```python
from build123d import *

# Parameters (mm, degrees)
BASE_FLANGE1_DEPTH     = 2
TAB1_START             = -2
TAB1_OUTLINE_W         = 950
TAB1_OUTLINE_H         = 35
TAB1_DEPTH             = 2
SKETCHED_START         = -950
SKETCHED_BEND1_DEPTH   = 950
SKETCHED_BEND1_2_DEPTH = 950
FILLET1_R              = 0.78
FILLET2_R              = 0.74
SKETCH10_R             = 12.5
SKETCH10_R_2           = 22.5
CUT_EXTRUDE1_DEPTH     = 10
SKETCH11_R             = 4
CUT_EXTRUDE2_DEPTH     = 10
SKETCH12_R             = 12.5
CUT_EXTRUDE3_DEPTH     = 10


# Read off the part's stored shape, not the designer's step: Tab1, Sketched Bend1
# Sheet-metal steps are written as plain solids
with BuildPart() as part:
    # Sketch1 → Base-Flange1 (new body)
    with BuildSketch(Plane(origin=(0, 0, 0), x_dir=(0, 0, -1), z_dir=(1, 0, 0))):
        Polygon((0, 0), (0, -300), (650, -550), (950, -550), (950, 0), align=None)
    extrude(amount=-BASE_FLANGE1_DEPTH)

    # Tab1 outline → Tab1 (add)
    with BuildSketch(Plane(origin=(0, 0, 0), x_dir=(0, 0, -1), z_dir=(1, 0, 0)).offset(TAB1_START)):
        with Locations((475, 17.5)):
            Rectangle(TAB1_OUTLINE_W, TAB1_OUTLINE_H)
    extrude(amount=TAB1_DEPTH)

    # Sketched Bend1 outline → Sketched Bend1 (cut)
    with BuildSketch(Plane.XY.offset(SKETCHED_START)):
        with BuildLine():
            ThreePointArc((-2, 0), (-1.443395312, 1.654267209), (0, 2.635602398))
            Line((0, 2.635602398), (0, 35))
            Line((0, 35), (-2, 35))
            Line((-2, 35), (-2, 0))
        make_face()
    extrude(amount=SKETCHED_BEND1_DEPTH, mode=Mode.SUBTRACT)

    # Sketched Bend1 2 outline → Sketched Bend1 2 (add)
    with BuildSketch(Plane.XY.offset(SKETCHED_START)):
        with BuildLine():
            Line((33.008755099, 2.7366), (0.7366, 2.7366))
            ThreePointArc((0.7366, 2.7366), (0.364854094, 2.711233029), (0, 2.635602398))
            Line((0, 2.635602398), (0, 0))
            ThreePointArc((0, 0), (0.215745145, 0.520854855), (0.7366, 0.7366))
            Line((0.7366, 0.7366), (33.008755099, 0.7366))
            Line((33.008755099, 0.7366), (33.008755099, 2.7366))
        make_face()
    extrude(amount=SKETCHED_BEND1_2_DEPTH)

    # Fillet1
    fillet1_edges = [part.edges().sort_by_distance(p)[0] for p in [
        (-1, -300, 0),
    ]]
    fillet(fillet1_edges, radius=FILLET1_R)

    # Fillet2
    fillet2_edges = [part.edges().sort_by_distance(p)[0] for p in [
        (-1, -550, -650),
    ]]
    fillet(fillet2_edges, radius=FILLET2_R)

    # Sketch10 → Cut-Extrude1 (cut)
    with BuildSketch(Plane(origin=(0, 0, 0), x_dir=(0, 0, -1), z_dir=(1, 0, 0))):
        with Locations((800.068700733, -27.5)):
            Circle(SKETCH10_R)
        with Locations((800.068700733, -522.5)):
            Circle(SKETCH10_R_2)
    extrude(amount=-CUT_EXTRUDE1_DEPTH, mode=Mode.SUBTRACT)

    # Sketch11 → Cut-Extrude2 (cut)
    with BuildSketch(Plane.XZ.offset(-0.7366)):
        with Locations((16.872677549, -25)):
            Circle(SKETCH11_R)
        with Locations((16.872677549, -125)):
            Circle(SKETCH11_R)
        with Locations((16.872677549, -225)):
            Circle(SKETCH11_R)
        with Locations((16.872677549, -325)):
            Circle(SKETCH11_R)
        with Locations((16.872677549, -425)):
            Circle(SKETCH11_R)
        with Locations((16.872677549, -525)):
            Circle(SKETCH11_R)
        with Locations((16.872677549, -625)):
            Circle(SKETCH11_R)
        with Locations((16.872677549, -725)):
            Circle(SKETCH11_R)
        with Locations((16.872677549, -825)):
            Circle(SKETCH11_R)
        with Locations((16.872677549, -925)):
            Circle(SKETCH11_R)
    extrude(amount=-CUT_EXTRUDE2_DEPTH, mode=Mode.SUBTRACT)

    # Sketch12 → Cut-Extrude3 (cut)
    with BuildSketch(Plane(origin=(0, 0, 0), x_dir=(0, 0, -1), z_dir=(1, 0, 0))):
        with Locations((125, -97.2634)):
            Circle(SKETCH12_R)
    extrude(amount=-CUT_EXTRUDE3_DEPTH, mode=Mode.SUBTRACT)


solid = part.part
```
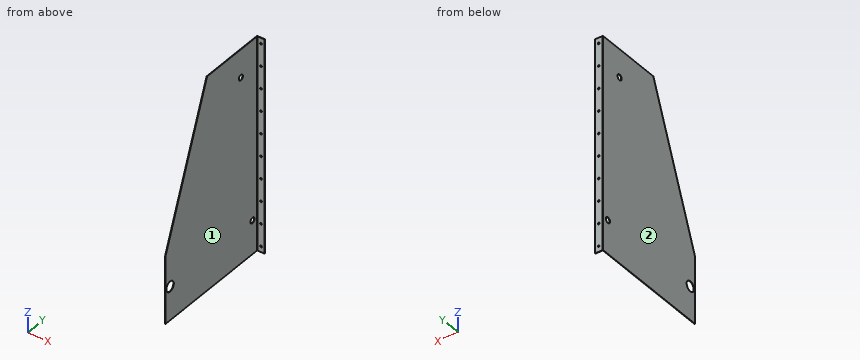
CAD build for the part. Positions are in the model's coordinates, mm. Face numbers are marked on the shaded views. Give positions to 0.01 mm unless a question says otherwise; leave off trailing zeros. Order: outer loops, then holes, each group sorted by start corner. A loop starts at its lowest first (then second) coordinate and runs counter-clockwise, first axis right, second up.
(1) Saw through at D-D, the plane y = -432. Give the cut face in (x, z), then the cut area to 3 significant figures.
(2) Flat gauge pins, fed straight in: pin 1 (2 mm diameter, centred on x = 3, z = -703, fed in from -Y); pin 2 (2 mm diameter, centred on y = -356.5, z = -327.5, fed in from +X); pin 3 (7 mm diameter, centred on x = 16.87, z = -525, fed in from +Y). Where does each tip first touch, or does it go through?
(3) Drill centre lines: L1, parallel to Y at x = 5, z = -229.5; L2, parallel to X at y = -274.5, z = -223; L3, parallel to Y at x = -1, z = -125 (3 decimals). Where is each one in solid material? Low to high.
(4) Mould opens along X. For the marked faces 1 and 2 say: released by +X, released by -X, zero draft, split by the parting line, or undercut.
(5) Saw through at B-B, the plane y = -309. Give the cut face in (x, z), then the cut area to 3 significant figures.
(6) Saw through at C-C, the plane z = -182.5. Give the cut face in (x, y), then the cut area to 3 significant figures.
(7) Saw through at A-A, the plane z = -665.5. Give the cut face in (x, y), then the cut area to 3 significant figures.
Results found:
1. outline: (-2, -950) - (0, -950) - (0, -343.2) - (-2, -343.2) - close
1. area: 1,210 mm2
2. pin 1: stops at y = 0.74
2. pin 2: stops at x = 0
2. pin 3: passes through
3. L1: y = 0.74 to 2.74
3. L2: x = -2 to 0
3. L3: y = -348.077 to -109.763, -84.763 to 2.115
4. face 1: released by +X
4. face 2: released by -X
5. outline: (-2, -950) - (0, -950) - (0, -23.4) - (-2, -23.4) - close
5. area: 1,850 mm2
6. outline: (-2, -370.19) - (0, -370.19) - (0, 0) arc R0.74 cw to (0.74, 0.74) - (33.01, 0.74) - (33.01, 2.74) - (0.74, 2.74) arc R2.74 ccw to (-2, 0) - close
6. area: 810 mm2
7. outline: (-2, -550) - (0, -550) - (0, 0) arc R0.74 cw to (0.74, 0.74) - (33.01, 0.74) - (33.01, 2.74) - (0.74, 2.74) arc R2.74 ccw to (-2, 0) - close
7. area: 1,170 mm2
